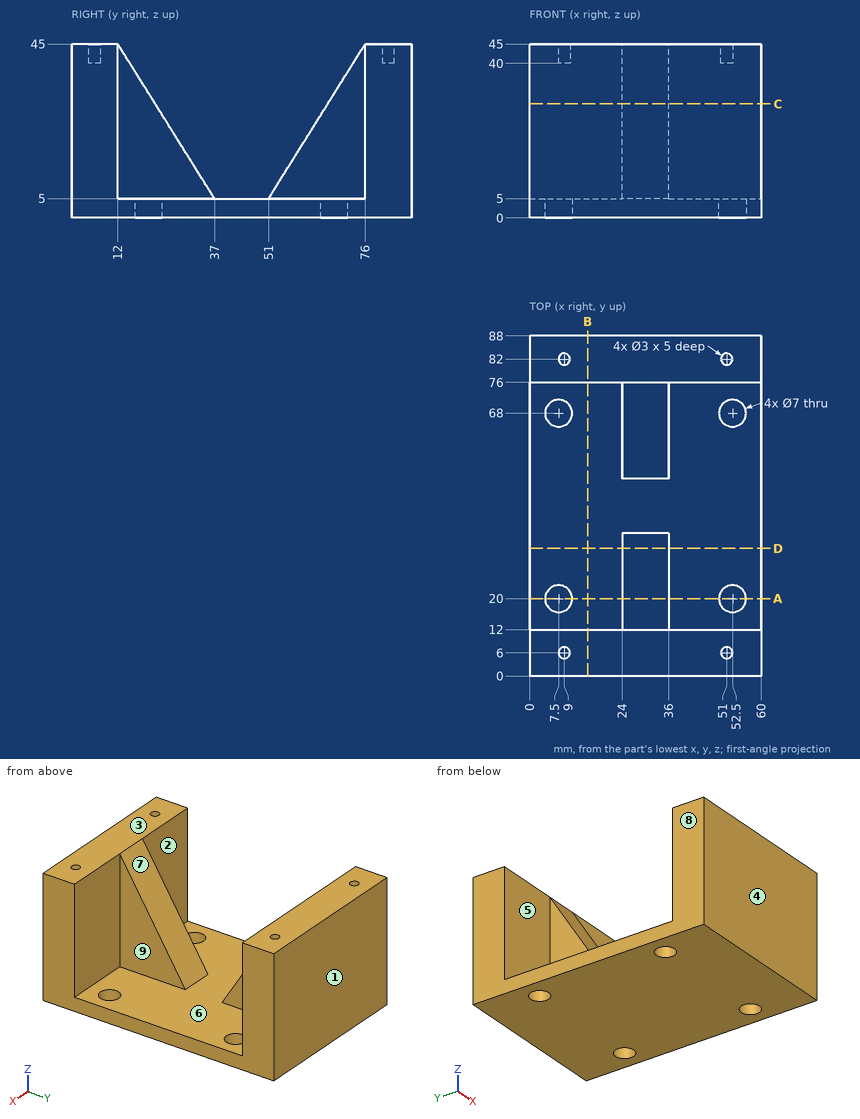
Source: three-view drawing plus pictorial views. Frame: mm from the lowest corner of the part. A direction names the side the tool comes from. Give positions to 0.01 mm unless a question says otherwise; leave off trailing zeros. Loops run counter-clockwise (first coordinate to the right, second up) from the corner with the lowest first, then second, coordinate; pieces in that order, holes last. Notation, with made-up numbers: (-29, 39) -> (-7, 39) arc R28 ccw to (-7, 63) -> close; hole circle Ø7 at (86.25, -15.5). An arc over 180 degrees is marked (long way). Put each result on its own line as item: value. Start each with the question number.
1) Material intervals for probe 1 along X at (y, z) = (82, 42); probe 2 along Y at (x, z) = (9, 41.25); probe 3 along Y at (x, z) = (7.5, 1.7), sorted ascending.
2) Contact query for flat-ended pins moving along their axis: P1, Ø20, axis at y = 63.5, z = 31, coming from the +X side; P2, Ø6, axis at x = 10.5, y = 63, coming from the +Z side; P3, Ø1.8, axis at x = 9, y = 82, coming from the +Z side. Output: stop coordinate, or through.
3) Cut plane D-D (y = 33). Return loops of the section in (x, z), then the cut area to 3 significant figures.
4) Cut plane B-B (x = 15). Return loops of the section in (y, z).
5) Cut plane A-A (y = 20). Return loops of the section in (x, z).
6) Draft query along Y for the marked faces 1, 2, 3 and 4. Return one class per face: released by +Y, released by -Y, zero draft, split by the parting line, or undercut.
7) Reachability of the marked faces 5, 6, 7, 8 and 9 from +Z, -Z, +X, -X, +Y, -Y: full face, straight path, thin tool, end or side. Return the list, or none.
8) Cut plane C-C (z = 29.5). Return loops of the section in (x, y), then the cut area to 3 significant figures.
Results are:
1. probe 1: x = 0 to 7.5, 10.5 to 49.5, 52.5 to 60
1. probe 2: y = 0 to 4.5, 7.5 to 12, 76 to 80.5, 83.5 to 88
1. probe 3: y = 0 to 16.5, 23.5 to 64.5, 71.5 to 88
2. P1: stops at x = 36
2. P2: stops at z = 5
2. P3: stops at z = 40
3. outline: (0, 0) -> (60, 0) -> (60, 5) -> (36, 5) -> (36, 11.4) -> (24, 11.4) -> (24, 5) -> (0, 5) -> close
3. area: 377 mm2
4. outline: (0, 0) -> (88, 0) -> (88, 45) -> (76, 45) -> (76, 5) -> (12, 5) -> (12, 45) -> (0, 45) -> close
5. outline: (0, 0) -> (4, 0) -> (4, 5) -> (0, 5) -> close; (11, 0) -> (49, 0) -> (49, 5) -> (36, 5) -> (36, 32.2) -> (24, 32.2) -> (24, 5) -> (11, 5) -> close; (56, 0) -> (60, 0) -> (60, 5) -> (56, 5) -> close
6. face 1: released by +Y
6. face 2: undercut
6. face 3: zero draft
6. face 4: released by -Y
7. face 5: +Z, -X
7. face 6: +Z
7. face 7: +Z, +X, -X
7. face 8: +Z, -Z, -X, +Y, -Y
7. face 9: +Z, +X
8. outline: (0, 0) -> (60, 0) -> (60, 12) -> (36, 12) -> (36, 21.69) -> (24, 21.69) -> (24, 12) -> (0, 12) -> close; (0, 76) -> (24, 76) -> (24, 66.31) -> (36, 66.31) -> (36, 76) -> (60, 76) -> (60, 88) -> (0, 88) -> close
8. area: 1,670 mm2
